Source: CAD feature listing. Evaluate the final solid. Frame: model axes, mm. Round coordinates to 2 decimals unless told otherwise and drop trailing zeros. Write each loop counter-clockwise with the first axis right and the second up, starting at its lowest first coordinate (ties: lowest second). Pieces come first, ordered by that corner, then holes. Notation, with made-up numbers: (-3.5, 19.5) -> (39.5, 19.5) arc R27 ccw to (39.5, 47.5) -> close; hole circle Ø6 at (44, 35.5). An arc over 180 degrees is marked (long way). Put each result on its own line as item: value.
```python
from build123d import *

# Parameters (mm, degrees)
SKETCH1_W           = 533.4
SKETCH1_H           = 152.4
BOSS_EXTRUDE1_DEPTH = 12.7
SKETCH2_W           = 25.4
SKETCH2_H           = 13.081
CUT_EXTRUDE1_DEPTH  = 555.889727784
SKETCH3_W           = 92.202
SKETCH3_H           = 13.081
CUT_EXTRUDE2_DEPTH  = 555.889727784


with BuildPart() as part:
    # Sketch1 → Boss-Extrude1 (new body)
    with BuildSketch(Plane.XY):
        with Locations((266.7, 76.2)):
            Rectangle(SKETCH1_W, SKETCH1_H)
    extrude(amount=BOSS_EXTRUDE1_DEPTH)

    # Sketch2 → Cut-Extrude1 (cut, through all)
    with BuildSketch(Plane.XY):
        with Locations((31.75, 31.9405)):
            Rectangle(SKETCH2_W, SKETCH2_H)
    extrude(amount=CUT_EXTRUDE1_DEPTH, mode=Mode.SUBTRACT)

    # Sketch3 → Cut-Extrude2 (cut, through all)
    with BuildSketch(Plane.XY):
        with Locations((236.601, 11.2903)):
            Rectangle(SKETCH3_W, SKETCH3_H)
    extrude(amount=CUT_EXTRUDE2_DEPTH, mode=Mode.SUBTRACT)


solid = part.part
```
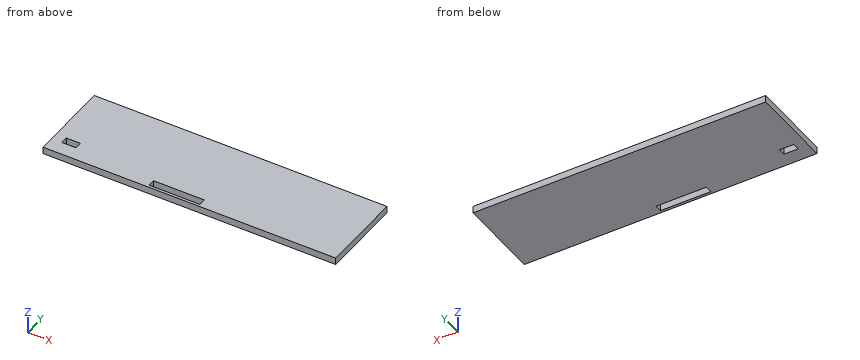
Q1. Material intervals for line 1 (Y direction, x = 274.5, z = 8.75); line 2 (X direction, y = 10, z = 9); line 3 (Y direction, x = 43.5, z = 8), sorted ascending. Write a range as [from, to].
Ans:
line 1: y = [0, 4.75], [17.83, 152.4]
line 2: x = [0, 190.5], [282.7, 533.4]
line 3: y = [0, 25.4], [38.48, 152.4]
Q2. Cut plane B-B on z = 4.25. Output: boundary loops of the cut face in (x, y).
Ans:
outline: (0, 0) -> (533.4, 0) -> (533.4, 152.4) -> (0, 152.4) -> close; hole (19.05, 25.4) -> (44.45, 25.4) -> (44.45, 38.48) -> (19.05, 38.48) -> close; hole (190.5, 4.75) -> (282.7, 4.75) -> (282.7, 17.83) -> (190.5, 17.83) -> close
Q3. Cut plane A-A on x = 205.5. Output: boundary loops of the cut face in (y, z), and give its area (3 significant figures).
Ans:
outline: (0, 0) -> (4.75, 0) -> (4.75, 12.7) -> (0, 12.7) -> close; (17.83, 0) -> (152.4, 0) -> (152.4, 12.7) -> (17.83, 12.7) -> close
area: 1,770 mm^2
